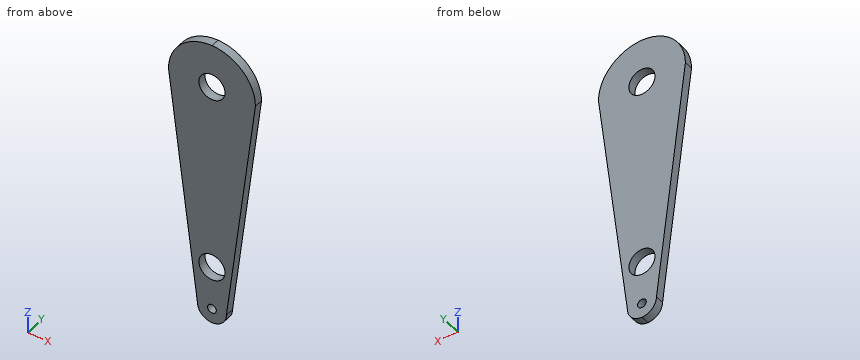
```python
from build123d import *

# Parameters (mm, degrees)
F0_R     = 1.5
F0_R_2   = 4.5
F1_DEPTH = 3


with BuildPart() as f1:
    # F0 (on Front) → F1 (new body)
    with BuildSketch(Plane.XZ):
        with BuildLine():
            ThreePointArc((-5, -45.000002), (-3.535534, -48.535536), (0, -50.000002))
            ThreePointArc((0, -50.000002), (3.535534, -48.535536), (5, -45.000002))
            Line((5, -45.000002), (15, 35))
            ThreePointArc((15, 35), (10.606602, 45.606602), (0, 50))
            ThreePointArc((0, 50), (-10.606602, 45.606602), (-15, 35))
            Line((-15, 35), (-5, -45.000002))
        make_face()
        with Locations((0, -45.000002)):
            Circle(F0_R, mode=Mode.SUBTRACT)
        with Locations((0, -30)):
            Circle(F0_R_2, mode=Mode.SUBTRACT)
        with Locations((0, 35)):
            Circle(F0_R_2, mode=Mode.SUBTRACT)
    extrude(amount=F1_DEPTH)


solid = f1.part
```
The listing builds one solid part. Answer for the finished solid, in the listing's coordinates (mm). Coordinates: 2 decimals unless noted, no trailing zeros. Write each loop counter-clockwise with the first axis right and the second up, starting at its lowest first coordinate (ties: lowest second). Pieces come first, ordered by that corner, then holes. Notation, with made-up numbers: (-4, -4) - (27, -4) arc R16 cw to (27, 19) - close; hole circle Ø3 at (21.5, -24.5). An arc over 180 degrees is marked (long way). Return JSON: item names as keys, results as strings. Group by question number.
Q1. The part is cut by section A-A on y = -1.45. Write down the section's boundary in (x, z), and give its area (3 significant figures).
Q2. Find the intervals of material crossed by line 1 along Z through (x, y) = (0, -2.05); line 2 along X through (y, z) = (-1.35, -45); line 3 along Z through (x, y) = (-1, -1.2), in increasing order. Write a range as [from, to].
Q3. The part is cut by section B-B on z = -30. Write down the section's boundary in (x, y) (3 decimals), and give its area (4 significant figures).
Q4. The part is cut by section C-C on z = -41. Write down the section's boundary in (x, y), and give its area (3 significant figures).
Q5. The part is cut by section D-D on x = 12. Write down the section's boundary in (y, z).
Q6. A flat-ended cylindrical pin translates along its axis: pin 1 Ø5 at (x, z) = (0, -45) entering from +Y. Find the tip coordinate at first contact, or state that the pin passes through.
Evaluation:
{
 "1": {"outline": "(-15, 35) - (-5, -45) arc R5 ccw to (5, -45) - (15, 35) arc R15 ccw to (0, 50) arc R15 ccw to start; hole circle Ø9 at (0, -30); hole circle Ø9 at (0, 35); hole circle Ø3 at (0, -45)", "area": "1,860 mm2"},
 "2": {"line 1": "z = [-50, -46.5], [-43.5, -34.5], [-25.5, 30.5], [39.5, 50]", "line 2": "x = [-5, -1.5], [1.5, 5]", "line 3": "z = [-49.9, -46.12], [-43.88, -34.39], [-25.61, 30.61], [39.39, 49.97]"},
 "3": {"outline": "(-6.875, -3) - (-4.5, -3) - (-4.5, 0) - (-6.875, 0) - close; (4.5, -3) - (6.875, -3) - (6.875, 0) - (4.5, 0) - close", "area": "14.25 mm2"},
 "4": {"outline": "(-5.5, -3) - (5.5, -3) - (5.5, 0) - (-5.5, 0) - close", "area": "33.0 mm2"},
 "5": {"outline": "(-3, 11) - (0, 11) - (0, 44) - (-3, 44) - close"},
 "6": {"pin 1": "stops at y = 0"}
}
